```python
from build123d import *

# Parameters (mm, degrees)
F1_DEPTH = 25.4
F2_DEPTH = 7.62
F3_DEPTH = 7.62


with BuildPart() as f1:
    # F0 (on Front) → F1 (new body)
    with BuildSketch(Plane.XZ):
        Polygon((-9.9045233801, -20.2733278275), (-44.2608483136, -20.2733278275), (-44.2608483136, -52.4630360305), (19.2391516864, -52.4630360305), (19.2391516864, -33.582534641), (-9.9045233801, -33.582534641), align=None)
    extrude(amount=-F1_DEPTH)

    # F2 (add): a face of the model
    f2_faces = [f1.faces().sort_by_distance(p)[0] for p in [
        (-27.0826858468, 12.7, -20.2733278275),
    ]]
    extrude(f2_faces, amount=F2_DEPTH)

    # F3 (add): a face of the model
    f3_faces = [f1.faces().sort_by_distance(p)[0] for p in [
        (-17.9738795934, 0, -35.5603880692),
    ]]
    extrude(f3_faces, amount=F3_DEPTH)


solid = f1.part
```
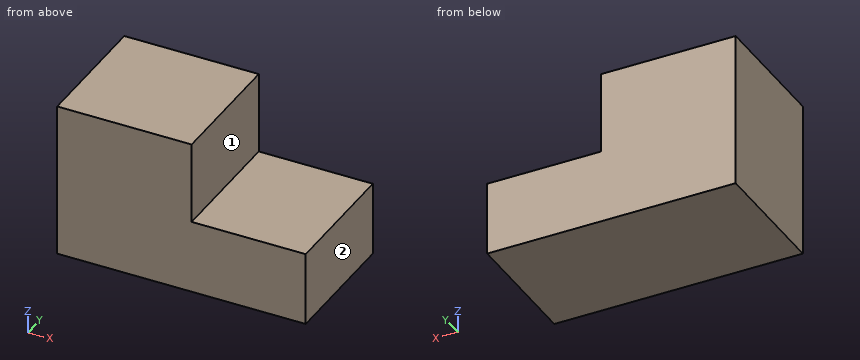
Input: part model. Units: mm. Frame: model coordinates. Face numbers are marked on the shaded views. A direction names the side the tool comes from. Coordinates: 2 decimals unless noted, no trailing zeros. Loops run counter-clockwise (first coordinate to the right, second up) from the corner with the lowest first, then second, coordinate; pieces in that order, holes last. Notation, with made-up numbers: (48.25, 44) -> (81.25, 44) arc R14 ccw to (81.25, 56) -> close; hole circle Ø1 at (-24, 85.25). An arc over 180 degrees is marked (long way). Use a Markdown table: item, result.
1) Cut plane B-B (x = -2). Return the cut outline in (y, z).
Results found:
| item | result |
|---|---|
| outline | (-7.62, -52.46) -> (25.4, -52.46) -> (25.4, -33.58) -> (-7.62, -33.58) -> close |
2) Cut plane A-A (y = -4). Return the cut outline in (x, z).
Results found:
| item | result |
|---|---|
| outline | (-44.26, -52.46) -> (19.24, -52.46) -> (19.24, -33.58) -> (-9.9, -33.58) -> (-9.9, -12.65) -> (-44.26, -12.65) -> close |
3) Contact query for a flat-ended pin moving along its axis: pin 1 (5 mm diameter, centred on x = -7, y = 5, fed in from +Z). Output: stop coordinate, or through.
Results found:
| item | result |
|---|---|
| pin 1 | stops at z = -33.58 |
4) Access query for the marked faces 1 and 2. Directions: +Z, -Z, +X, -X, +Y, -Y. A direction counts if a zero-diameter tool reaches every point of the face in a straight line with its end or side. Return the directions, or none.
Results found:
| item | result |
|---|---|
| face 1 | +Z, +X, +Y, -Y |
| face 2 | +Z, -Z, +X, +Y, -Y |
5) Material intervals for line 1 along X through (y, z) = (3, -33.5); line 2 along Z through (x, y) = (3, 1.5), sorted ascending. Write a range as from..to.
Results found:
| item | result |
|---|---|
| line 1 | x = -44.26..-9.9 |
| line 2 | z = -52.46..-33.58 |
6) Cut plane C-C (z = -30). Return the cut outline in (x, y), then the cut area to 3 significant figures.
Results found:
| item | result |
|---|---|
| outline | (-44.26, -7.62) -> (-9.9, -7.62) -> (-9.9, 25.4) -> (-44.26, 25.4) -> close |
| area | 1,130 mm2 |
